Verification items for the finished model (mm, model axes). Coordinates: 2 decimals unless noted, no trailing zeros. Order: outer loops, then holes, each group sorted by start corner. A loop starts at its lowest first (then second) coordinate and runs counter-clockwise, first axis right, second up. Notation, with made-up numbers: M 28.5,70 L 55.5,70 A36 cw 55.5,109 Z; hole C -40,31.5 d4. An arc over 180 degrees is marked long. Write item = value, one per line.
```python
from build123d import *

# Parameters (mm, degrees)
F0_W      = 300
F0_H      = 400
F1_DEPTH  = 19
F2_W      = 280
F2_H      = 380
F3_DEPTH  = 2
F4_W      = 260
F4_H      = 358
F5_DEPTH  = 17
F6_SIZE   = 5
F7_W      = 10
F7_H      = 80
F8_DEPTH  = 17
F9_W      = 10
F9_H      = 80
F10_DEPTH = 17


with BuildPart() as f1:
    # F0 (on Front) → F1 (new body)
    with BuildSketch(Plane.XZ):
        with Locations((-31.717002, 227.192586)):
            Rectangle(F0_W, F0_H)
    extrude(amount=F1_DEPTH)

    # F2 (on face) → F3 (cut)
    with BuildSketch(Plane(origin=(0, 0, 0), x_dir=(-1, 0, 0), z_dir=(0, 1, 0))):
        with Locations((31.717002, 227.192586)):
            Rectangle(F2_W, F2_H)
    extrude(amount=-F3_DEPTH, mode=Mode.SUBTRACT)

    # F4 (on face) → F5 (cut)
    with BuildSketch(Plane(origin=(0, -2, 0), x_dir=(-1, 0, 0), z_dir=(0, 1, 0))):
        with Locations((31.717002, 228.192586)):
            Rectangle(F4_W, F4_H)
    extrude(amount=-F5_DEPTH, mode=Mode.SUBTRACT)

    # F6
    f6_edges = [f1.edges().sort_by_distance(p)[0] for p in [
        (118.282998, 0, 227.192586),
        (-181.717002, 0, 227.192586),
    ]]
    chamfer(f6_edges, length=F6_SIZE)

    # F7 (on face) → F8 (cut)
    with BuildSketch(Plane(origin=(0, -2, 0), x_dir=(-1, 0, 0), z_dir=(0, 1, 0))):
        with Locations((-103.282998, 97.192586)):
            Rectangle(F7_W, F7_H)
    extrude(amount=-F8_DEPTH, mode=Mode.SUBTRACT)

    # F9 (on face) → F10 (cut)
    with BuildSketch(Plane(origin=(0, -2, 0), x_dir=(-1, 0, 0), z_dir=(0, 1, 0))):
        with Locations((166.717002, 97.192586)):
            Rectangle(F9_W, F9_H)
    extrude(amount=-F10_DEPTH, mode=Mode.SUBTRACT)


solid = f1.part
```
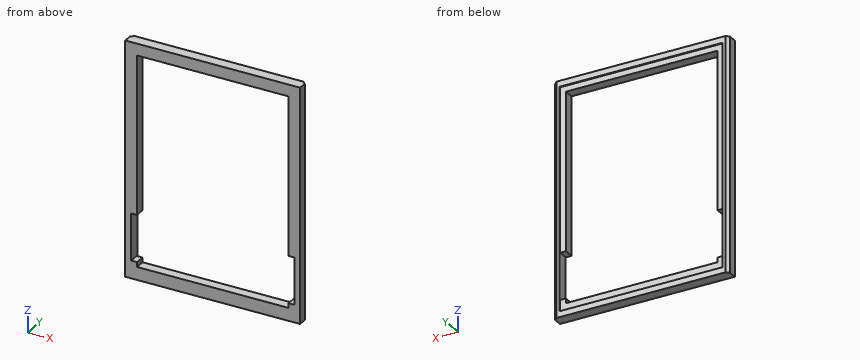
Item 1: Sectioned sample at B-B, the plane z = 280.5. Enter the section's corners in (x, y).
Report:
outline = M -181.72,-19 L -161.72,-19 L -161.72,-2 L -171.72,-2 L -171.72,0 L -176.72,0 L -181.72,-5 Z; M 98.28,-19 L 118.28,-19 L 118.28,-5 L 113.28,0 L 108.28,0 L 108.28,-2 L 98.28,-2 Z
Item 2: Sectioned sample at D-D, the plane z = 109.5. Enter the section's corners in (x, y), then the cut area to 3 significant figures.
Report:
outline = M -181.72,-19 L -171.72,-19 L -171.72,0 L -176.72,0 L -181.72,-5 Z; M 108.28,-19 L 118.28,-19 L 118.28,-5 L 113.28,0 L 108.28,0 Z
area = 355 mm^2
Item 3: Sectioned sample at A-A, the plane x = 81.5. Enter the section's corners in (y, z).
Report:
outline = M -19,27.19 L 0,27.19 L 0,37.19 L -2,37.19 L -2,49.19 L -19,49.19 Z; M -19,407.19 L -2,407.19 L -2,417.19 L 0,417.19 L 0,427.19 L -19,427.19 Z
Item 4: Gauge pin test, flat end, axial feed: pin 1 (6 mm diameter, centred on x = -100.5, z = 49, fed in from +Y). Record the tip position at first contact, or that the pin passes through.
Report:
pin_1 = -2
Item 5: Scan lines: L1, parallel to Z at x = -131.5, y = -6; L2, parallel to X at y = -5, z = 361; L3, parallel to X at y = -7.5, z = 63.5. Record each from-to range of solid material in increasing order. Write a range as from..to.
Report:
L1 = 27.19..49.19, 407.19..427.19
L2 = -181.72..-161.72, 98.28..118.28
L3 = -181.72..-171.72, 108.28..118.28
Item 6: Sectioned sample at C-C, the plane y = -9.5. Enter the section's corners in (x, z).
Report:
outline = M -181.72,27.19 L 118.28,27.19 L 118.28,427.19 L -181.72,427.19 Z; hole M -171.72,57.19 L -161.72,57.19 L -161.72,49.19 L 98.28,49.19 L 98.28,57.19 L 108.28,57.19 L 108.28,137.19 L 98.28,137.19 L 98.28,407.19 L -161.72,407.19 L -161.72,137.19 L -171.72,137.19 Z
